For this review, take the finished solid that the model builds, in its own axes (mm). Give positions to 0.01 mm unless a question says otherwise; leave off trailing zeros. Loops run counter-clockwise (first coordinate to the right, second up) from the corner with the lowest first, then second, coordinate; pieces in that order, holes last. Notation, with made-up numbers: M 34.25,53 L 66.25,53 A24 ccw 66.25,87 Z; hole C 72.25,69.25 d8. An arc over 180 degrees is marked long. Use CSV: the item, a comma, the result in double quotes. Start each with the question number.
1. Take a section at A-A, the plane y = 0. Write out the cut boundary in (x, z).
2. The part is to be moulded in two halves that separate along X. For faces 1 (the face through (2.75, 12.4, 90.14)), 2 (the face through (-40.409, -30.985, 87.833)), 3 (the face through (16, 1, 177.8)), say which applies: pulls with the +X half, pulls with the -X half, needs draft (parallel to the pull), parting line crosses it, or undercut.
3. Take a section at C-C, the plane z = 123.5. Write out the cut boundary in (x, y), and give its area (3 significant figures).
4. To check wall thickness, follow line 1 (Y direction, x = 0, z = 46); line 2 (X direction, y = -4, z = 35); line 3 (X direction, y = -5, z = 14). State the ranges of each line that lie inside material, in increasing order. Write a range as [from, to].
5. Insertion check: P1, Ø6, axis at x = 3.5, y = 39, coming from the -Z side; P2, Ø12, axis at y = 15.5, z = 21.5, coming from the +X side; P3, Ø2, axis at x = 0.5, z = 96.5, coming from the +Y side; P4, Ø1, axis at x = -22, z = 137, coming from the -Y side. Each pin has a flat end and moves straight along its axis. Give the tip position at first contact, or say it passes through.
from build123d import *

# Parameters (mm, degrees)
F0_R     = 50.921014
F1_DEPTH = 177.8
F2_R     = 12.7
F5_D     = 25.4
F5_DEPTH = 177.8


with BuildPart() as f1:
    # F0 (on Top) → F1 (new body)
    with BuildSketch(Plane.XY):
        Circle(F0_R)
    extrude(amount=F1_DEPTH)

    # F2
    f2_edges = [f1.edges().sort_by_distance(p)[0] for p in [
        (-50.921014, 0, 0),
        (-50.921014, 0, 177.8),
    ]]
    fillet(f2_edges, radius=F2_R)

    # F5
    with Locations(Plane(origin=(0, 0, 0), x_dir=(1, 0, 0), z_dir=(0, 0, -1))):
        with Locations((0, 0)):
            Hole(F5_D / 2, depth=F5_DEPTH)


solid = f1.part
Result set:
1,outline,"M -50.92,12.7 A12.7 ccw -38.22,0 L -12.7,0 L -12.7,177.8 L -38.22,177.8 A12.7 ccw -50.92,165.1 Z; M 12.7,0 L 38.22,0 A12.7 ccw 50.92,12.7 L 50.92,165.1 A12.7 ccw 38.22,177.8 L 12.7,177.8 Z"
2,face 1,"undercut"
2,face 2,"parting line crosses it"
2,face 3,"needs draft"
3,outline,"C 0,0 d101.84; hole C 0,0 d25.4"
3,area,"7,640 mm2"
4,line 1,"[-50.92, -12.7], [12.7, 50.92]"
4,line 2,"[-50.76, -12.05], [12.05, 50.76]"
4,line 3,"[-50.67, -11.67], [11.67, 50.67]"
5,P1,"z = 0"
5,P2,"x = 50.03"
5,P3,"y = 50.92"
5,P4,"y = -46.16"
